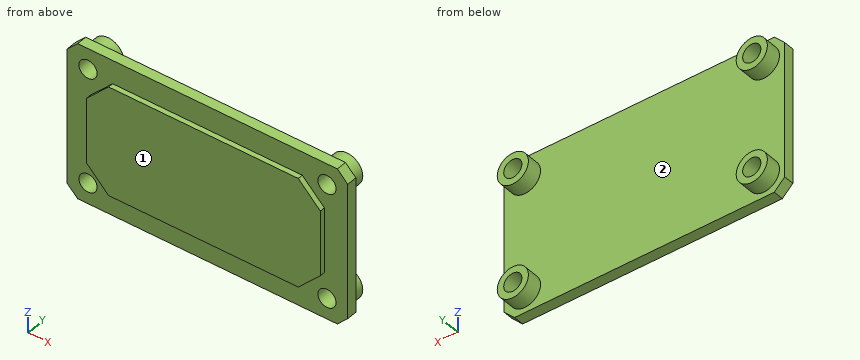
```python
from build123d import *

# Parameters (mm, degrees)
F3_W      = 85.725
F3_H      = 47.625
F4_DEPTH  = 3.175
F6_DEPTH  = 1.5875
F7_R      = 4.7625
F8_DEPTH  = 7.9375
F9_R      = 2.778125
F10_DEPTH = 7.9375
F11_SIZE  = 3.175


with BuildPart() as f4:
    # F3 (on Front) → F4 (new body, through all)
    with BuildSketch(Plane.XZ):
        Rectangle(F3_W, F3_H)
    extrude(amount=-F4_DEPTH)

    # F5 (on Front) → F6 (join)
    with BuildSketch(Plane.XZ):
        Polygon((28.98775, 16.66875), (-28.98775, 16.66875), (-35.71875, 9.93775), (-35.71875, -9.93775), (-28.98775, -16.66875), (28.98775, -16.66875), (35.71875, -9.93775), (35.71875, 9.93775), align=None)
    extrude(amount=F6_DEPTH)

    # F7 (on Front) → F8 (join)
    with BuildSketch(Plane.XZ):
        with Locations((36.5125, 17.4625)):
            Circle(F7_R)
        with Locations((-36.5125, 17.4625)):
            Circle(F7_R)
        with Locations((-36.5125, -17.4625)):
            Circle(F7_R)
        with Locations((36.5125, -17.4625)):
            Circle(F7_R)
    extrude(amount=-F8_DEPTH)

    # F9 (on Front) → F10 (cut, through all)
    with BuildSketch(Plane.XZ):
        with Locations((36.5125, 17.4625)):
            Circle(F9_R)
        with Locations((36.5125, -17.4625)):
            Circle(F9_R)
        with Locations((-36.5125, 17.4625)):
            Circle(F9_R)
        with Locations((-36.5125, -17.4625)):
            Circle(F9_R)
    extrude(amount=-F10_DEPTH, mode=Mode.SUBTRACT)

    # F11
    f11_edges = [f4.edges().sort_by_distance(p)[0] for p in [
        (42.8625, 1.5875, -23.8125),
        (42.8625, 1.5875, 23.8125),
        (-42.8625, 1.5875, -23.8125),
        (-42.8625, 1.5875, 23.8125),
    ]]
    chamfer(f11_edges, length=F11_SIZE)


solid = f4.part
```
Here's how the part is built. I have some questions about the finished solid (model axes, mm). Face numbers are marked on the shaded views. Coordinates: 2 decimals unless noted, no trailing zeros. Loops run counter-clockwise (first coordinate to the right, second up) from the corner with the lowest first, then second, coordinate; pieces in that order, holes last. Notation, with made-up numbers: M -18.75,76 L 32.25,76 A17 cw 32.25,105 Z; hole C 24.5,-18 d10. An arc over 180 degrees is marked long. One line per item, written item: value.
1. Imagine slicing it at A-A (z = -18.5). List the corners of the cut face in (x, y) for me (1 decimal), and give its area (3 significant figures).
Geometry says:
outline: M -42.9,0 L -39.1,0 L -39.1,7.9 L -41.2,7.9 L -41.2,3.2 L -42.9,3.2 Z; M -33.9,0 L 33.9,0 L 33.9,7.9 L 31.9,7.9 L 31.9,3.2 L -31.9,3.2 L -31.9,7.9 L -33.9,7.9 Z; M 39.1,0 L 42.9,0 L 42.9,3.2 L 41.2,3.2 L 41.2,7.9 L 39.1,7.9 Z
area: 279 mm2
2. Imagine slicing it at C-C (y = 1.5). List the corners of the cut face in (x, z) for me, and give its area (3 significant figures).
Geometry says:
outline: M -42.86,-20.64 L -39.69,-23.81 L 39.69,-23.81 L 42.86,-20.64 L 42.86,20.64 L 39.69,23.81 L -39.69,23.81 L -42.86,20.64 Z; hole C -36.51,-17.46 d5.56; hole C -36.51,17.46 d5.56; hole C 36.51,-17.46 d5.56; hole C 36.51,17.46 d5.56
area: 3,970 mm2
3. Imagine slicing it at B-B (x = -5.5). List the corners of the cut face in (y, z) for me (1 decimal).
Geometry says:
outline: M -1.6,-16.7 L 0,-16.7 L 0,-23.8 L 3.2,-23.8 L 3.2,23.8 L 0,23.8 L 0,16.7 L -1.6,16.7 Z
4. Please list where these lines run through material, in increasing order: probe 1 along X at (y, z) = (0.25, -16.5); probe 2 along Y at (x, z) = (-19.5, -16) (1 decimal); probe 3 along Y at (x, z) = (-14, -18) (3 decimals).
Geometry says:
probe 1: x = -42.86 to -39.12, -33.91 to 33.91, 39.12 to 42.86
probe 2: y = -1.6 to 3.2
probe 3: y = 0 to 3.175
5. Thinking about a two-plate mould opening in X: for the marked faces 1 and 2, which applies, +X half, -X half, draft (parallel to the pull), parting line (faces both ways), or undercut?
Geometry says:
face 1: draft
face 2: undercut
6. Will these pins go through, and if not, where does the flat tip stop? pin 1 Ø6.5 at (x, z) = (-36.51, -17.46) entering from -Y; pin 2 Ø5 at (x, z) = (36.51, -17.46) entering from +Y; pin 3 Ø12 at (x, z) = (11, -1) entering from +Y (3 decimals); pin 4 Ø1 at (y, z) = (5, -14) entering from +X.
Geometry says:
pin 1: stops at y = 0
pin 2: passes through
pin 3: stops at y = 3.175
pin 4: stops at x = 40.24
7. Imagine slicing it at D-D (z = 0.5). List the corners of the cut face in (x, y) for me (1 decimal).
Geometry says:
outline: M -42.9,0 L -35.7,0 L -35.7,-1.6 L 35.7,-1.6 L 35.7,0 L 42.9,0 L 42.9,3.2 L -42.9,3.2 Z
